Autodesk Inventor part; units mm, degrees
ref_plane "YZ Plane" through (0, 0, 0) normal (1, 0, 0) x (0, 1, 0)
ref_plane "XZ Plane" through (0, 0, 0) normal (0, 1, 0) x (-1, 0, 0)
ref_plane "XY Plane" through (0, 0, 0) normal (0, 0, 1) x (1, 0, 0)
sketch "Sketch1" plane through (0, 0, 0) normal (0, 0, 1) x (1, 0, 0)
  line L0 (0, 0) -> (8.7313, 0) construction
  line L1 (0, 0) -> (0, 7.9375) construction
  line L2 (0, 7.9375) -> (8.7312, 7.9375) construction
  line L3 (8.7312, 7.9375) -> (8.7313, 0) construction
  line L4 (8.7312, 7.9375) -> (47.625, 7.9375) construction
  line L5 (8.7312, 7.9375) -> (8.7312, 14.2875) construction
  line L6 (8.7312, 14.2875) -> (11.9062, 14.2875) construction
  line L7 (11.9062, 14.2875) -> (11.9062, 0) construction
  line L8 (11.9062, 0) -> (8.7313, 0) construction
  line L9 (11.9062, 0) -> (21.4312, 0) construction
  line L10 (21.4312, 0) -> (21.4312, 26.67) construction
  line L11 (21.4312, 26.67) -> (11.9063, 26.67) construction
  line L12 (11.9063, 26.67) -> (11.9062, 14.2875) construction
  line L13 (16.6687, 0) -> (16.6687, 26.67) construction
  line L14 (16.6687, 17.4625) -> (23.8125, 17.4625) construction
  line L15 (23.8125, 17.4625) -> (23.8125, 0) construction
  line L16 (23.8125, 0) -> (21.4312, 0) construction
  line L17 (23.8125, 0) -> (24.6062, 0) construction
  line L18 (24.6062, 0) -> (24.6062, 14.2875) construction
  line L19 (24.6062, 14.2875) -> (23.8125, 14.2875) construction
  line L20 (23.8125, 14.2875) -> (23.8125, 0) construction
  line L21 (24.6062, 0) -> (34.1312, 0) construction
  line L22 (34.1312, 0) -> (34.1313, 20.32) construction
  line L23 (34.1313, 20.32) -> (24.6062, 20.32) construction
  line L24 (24.6062, 20.32) -> (24.6062, 0) construction
  line L25 (29.3687, 20.32) -> (29.3687, 0) construction
  line L26 (29.3687, 17.4625) -> (36.5125, 17.4625) construction
  line L27 (36.5125, 17.4625) -> (36.5125, 0) construction
  line L28 (36.5125, 0) -> (34.1312, 0) construction
  line L29 (36.5125, 0) -> (37.3062, 0) construction
  line L30 (37.3062, 0) -> (37.3062, 14.2875) construction
  line L31 (37.3062, 14.2875) -> (36.5125, 14.2875) construction
  line L32 (36.5125, 14.2875) -> (36.5125, 0) construction
  line L33 (37.3062, 0) -> (38.8937, 0) construction
  line L34 (38.8937, 0) -> (38.8937, 9.525) construction
  line L35 (38.8937, 9.525) -> (37.3062, 9.525) construction
  line L36 (37.3062, 9.525) -> (37.3062, 0) construction
  line L37 (47.625, 7.9375) -> (47.625, 0) construction
  line L38 (47.625, 0) -> (38.8937, 0) construction
  line L39 (14.2875, 26.67) -> (14.2875, 0) construction
  line L40 (26.9875, 20.32) -> (26.9875, 0) construction
  line L41 (0, 7.9375) -> (0, 17.4625) construction
  line L42 (0, 17.4625) -> (8.7312, 17.4625) construction
  line L43 (8.7312, 17.4625) -> (8.7312, 14.2875) construction
  line L44 (0, 3.175) -> (47.625, 3.175) construction
  circle A0 centre (14.2875, 5.5563) radius 2.3813 construction
  circle A1 centre (26.9875, 5.5562) radius 2.3812 construction
  circle A2 centre (14.2875, 5.8102) radius 2.3813 construction
  circle A3 centre (14.2875, 7.5565) radius 2.3813 construction
  circle A4 centre (26.9875, 5.8103) radius 2.3812 construction
  circle A5 centre (26.9875, 7.5565) radius 2.3812 construction
  line L45 (11.9062, 8.1915) -> (16.6687, 8.1915) construction
  line L46 (15.0198, 3.175) -> (17.0201, 5.1753) construction
  line L47 (17.0201, 5.1753) -> (24.2549, 5.1753) construction
  line L48 (24.2549, 5.1753) -> (26.2552, 3.175) construction
  line L49 (24.6062, 8.1915) -> (29.3687, 8.1915) construction
  line L50 (12.7, 5.1753) -> (19.8713, 5.1753) construction
  line L51 (28.575, 5.1753) -> (21.4037, 5.1753)
  line L52 (0, 6.35) -> (9.1122, 6.35) construction
  line L53 (9.1122, 6.35) -> (9.1122, 0) construction
  line L54 (12.7, 5.1753) -> (10.6997, 3.175) construction
  line L55 (19.8713, 5.1753) -> (21.8716, 3.175) construction
  line L56 (21.8716, 3.175) -> (28.575, 3.175) construction
  line L57 (28.575, 3.175) -> (30.4827, 0) construction
  line L58 (28.575, 5.1753) -> (30.5753, 3.175)
  line L59 (30.5753, 3.175) -> (37.2787, 3.175)
  line L60 (37.2787, 3.175) -> (39.1864, 0)
  line L61 (9.1122, 5.5562) -> (47.625, 5.5563) construction
  line L62 (39.5833, 0) -> (36.2448, 5.5563) construction
  line L63 (21.4037, 5.1753) -> (19.4034, 3.175)
  line L64 (19.4034, 3.175) -> (-3.0861, 3.175)
  line L65 (47.625, 7.9375) -> (47.625, 17.4625) construction
  line L66 (47.625, 17.4625) -> (38.8937, 17.4625) construction
  line L67 (38.8937, 17.4625) -> (38.8937, 9.525) construction
  line L68 (47.625, 7.9375) -> (53.975, 7.9375) construction
  line L69 (53.975, 7.9375) -> (53.975, 0) construction
  line L70 (53.975, 0) -> (47.625, 0) construction
  line L71 (53.975, 6.35) -> (66.675, 6.35) construction
  line L72 (66.675, 6.35) -> (66.675, 0) construction
  line L73 (66.675, 0) -> (53.975, 0) construction
  line L74 (-8.0645, 3.175) -> (-8.0645, 2.3812) construction
  line L75 (-8.0645, 0) -> (39.1864, 0)
  line L76 (-3.0861, 3.175) -> (-3.0861, 2.3812)
  line L77 (-3.0861, 2.3812) -> (-8.0645, 2.3812)
  line L78 (-8.0645, 3.175) -> (-8.0645, 6.35) construction
  line L79 (-8.0645, 6.35) -> (-3.0861, 6.35) construction
  line L80 (-3.0861, 6.35) -> (-3.0861, 3.175) construction
  line L81 (-3.0861, 0) -> (-3.0861, 2.3812) construction
  line L82 (-1.5875, 0) -> (-1.5875, 11.1125) construction
  line L83 (-1.5875, 11.1125) -> (-3.0861, 11.1125) construction
  line L84 (-3.0861, 11.1125) -> (-3.0861, 6.35) construction
  line L85 (-3.0861, 3.175) -> (-8.0645, 3.175) construction
  line L86 (-8.0645, 2.3812) -> (-8.0645, 0) construction
  line L87 (-8.0645, 2.7051) -> (-9.5631, 2.7051) construction
  line L88 (-9.5631, 2.7051) -> (-9.5631, 0) construction
  line L89 (-9.5631, 0) -> (-8.0645, 0) construction
  line L90 (-8.0645, 1.4224) -> (-5.5245, 1.4224) construction
  line L91 (-5.5245, 1.4224) -> (-5.5245, 0) construction
  line L92 (-5.5245, 1.4224) -> (-2.9845, 1.4224) construction
  line L93 (-2.9845, 1.4224) -> (-2.9845, 0) construction
  line L94 (-3.0861, 11.1125) -> (-14.2875, 11.1125) construction
  line L95 (-14.2875, 11.1125) -> (-14.2875, 5.9531) construction
  line L96 (-14.2875, 5.9531) -> (-18.4912, 5.9531) construction
  line L97 (-18.4912, 5.9531) -> (-18.4912, 0) construction
  line L98 (-18.4912, 0) -> (-9.5631, 0) construction
  line L99 (-8.0645, 3.9687) -> (-14.5224, 3.9687) construction
  line L100 (-14.5224, 3.9687) -> (-14.5224, 0) construction
  line L101 (-14.5224, 3.429) -> (-10.3568, 3.429) construction
  line L102 (-10.3568, 3.429) -> (-10.3568, 0) construction
  line L103 (-16.9037, 3.175) -> (-16.9037, 0) construction
  line L104 (-16.9037, 3.175) -> (-18.4912, 3.175) construction
  dimension "d0" = 8.7312
  dimension "d1" = 7.9375
  dimension "d2" = 3.175
  dimension "d3" = 14.2875
  dimension "d4" = 9.525
  dimension "d5" = 26.67
  dimension "d6" = 7.1437
  dimension "d7" = 17.4625
  dimension "d8" = 0.7937
  dimension "d9" = 14.2875
  dimension "d10" = 9.525
  dimension "d11" = 20.32
  dimension "d12" = 7.1437
  dimension "d13" = 17.4625
  dimension "d14" = 0.7937
  dimension "d15" = 14.2875
  dimension "d16" = 1.5875
  dimension "d17" = 9.525
  dimension "d18" = 8.7312
  dimension "d19" = 2.3813
  dimension "d20" = 2.3813
  dimension "d21" = 17.4625
  dimension "d22" = 3.175
  dimension "d23" = 4.7625
  dimension "d24" = 4.7625
  dimension "d26" = 0.254
  dimension "d28" = 45
  dimension "d29" = 45
  dimension "d30" = 0.254
  dimension "d31" = 7.2348
  dimension "d32" = 5.1753
  dimension "d33" = 7.1713
  dimension "d34" = 1.5875
  dimension "d35" = 7.1713
  dimension "d36" = 1.5875
  dimension "d37" = 6.35
  dimension "d39" = 45
  dimension "d40" = 45
  dimension "d41" = 1.5875
  dimension "d42" = 59
  dimension "d43" = 6.7034
  dimension "d44" = 6.7034
  dimension "d45" = 5.5563
  dimension "d46" = 0.3969
  dimension "d47" = 1.5875
  dimension "d48" = 9.1122
  dimension "d52" = 17.4625
  dimension "d53" = 6.35
  dimension "d54" = 12.7
  dimension "d55" = 6.35
  dimension "d56" = 2.3813
  dimension "d57" = 4.9784
  dimension "d58" = 6.35
  dimension "d66" = 1.4986
  dimension "d67" = 1.5875
  dimension "d68" = 11.1125
  dimension "d69" = 2.7051
  dimension "d70" = 1.4986
  dimension "d71" = 1.4224
  dimension "d72" = 2.54
  dimension "d73" = 2.54
  dimension "d74" = 3.9688
  dimension "d75" = 4.1656
  dimension "d76" = 3.429
sketch "Sketch2" plane through (0, 0, 0) normal (0, 0, 1) x (1, 0, 0)
  line L0 (19.4034, 3.175) -> (-3.0861, 3.175)
  line L1 (-3.0861, 3.175) -> (-3.0861, 2.3812)
  line L2 (-3.0861, 2.3812) -> (-8.0645, 2.3812)
  line L3 (-8.0645, 2.3812) -> (-8.0645, 0)
  line L4 (-8.0645, 0) -> (39.1864, 0)
  line L5 (37.2787, 3.175) -> (39.1864, 0)
  line L6 (30.5753, 3.175) -> (37.2787, 3.175)
  line L7 (28.575, 5.1753) -> (30.5753, 3.175)
  line L8 (28.575, 5.1753) -> (21.4037, 5.1753)
  line L9 (21.4037, 5.1753) -> (19.4034, 3.175)
  point P0 (0, 0)
revolve "Revolution1" add sketch "Sketch2" angle 360 about axis through (-8.0645, 0, 0) along (1, 0, 0)
sketch "Sketch3" plane through (-8.0645, 0, 0) normal (-1, 0, 0) x (0, 0, 1)
  circle A0 centre (0, 0) radius 2.3813
hole "Hole1" at (-8.0645, 0, 0) direction (1, 0, 0) diameter 2.159 depth 3.81 tip angle 118
equation "\"d9\" = d3"
equation "\"d12\" = d6"
equation "\"d13\" = d7"
equation "\"d15\" = d9"
equation "\"d18\" = d0"
equation "\"d20\" = d19"
equation "\"d35\" = d33"
equation "\"d36\" = d34"
equation "\"d43\" = d44"
equation "\"d52\" = d13"
properties part number "Ball Shifting Outline" material "Steel, Alloy"
Input: part model. Units: mm. Frame: model coordinates. A direction names the side the tool comes from. Give positions to 0.01 mm unless a question says otherwise; leave off trailing zeros. Write each loop counter-clockwise with the first axis right and the second up, starting at its lowest first coordinate (ties: lowest second). Pieces come first, ordered by that corner, then holes. Notation, with made-up numbers: M 10.5,60.25 L 58.5,60.25 A10 ccw 58.5,76.25 Z; hole C -5.75,17.25 d6. An arc over 180 degrees is marked long. Write item = value, one per line. Start each with the question number.
1) Reachability of faces 1 (the cylindrical face through (-5.61, -0.516, 2.325)), 2 (the cylindrical face through (24.94, -0.67, -5.13)), 3 (the cylindrical face through (33.97, -0.69, -3.1)) from +Z, -Z, +X, -X, +Y, -Y: full face, straight path, thin tool, end or side. Return the list, or none.
2) Draft query along Y for faces 4 (the flat face through (-8.065, 1, 1)), 5 (the cylindrical face through (-6.13, -1.07, -0.14)), 6 (the cylindrical face through (8, -0.69, 3.1)), 7 (the conical face through (-3.719, -0.183, -0.041)). Return one class per face: +Y half, -Y half, draft (parallel to the pull), parting line (faces both ways), or undercut.
3) Cut plane A-A on x = 12. Return the cut outline in (y, z) (3 decimals), then the cut area to 3 significant figures.
4) Material intervals for line 1 along Z through (x, y) = (-5.6, 0); line 2 along X through (y, z) = (-3.5, -3); line 3 along Z through (x, y) = (10.5, 1.5), sorted ascending. Write a range as [from, to].
5) First-contact query: pin 1 Ø3 at (x, z) = (25.5, -1.5) entering from +Y; pin 2 Ø3 at (x, z) = (23.5, -3) entering from -Y; pin 3 Ø1.5 at (y, z) = (0.5, 1) entering from +X; pin 4 Ø4 at (x, z) = (5, -1.5) entering from -Y (3 decimals). Flat tips, straight axial feed; report the tip coordinate or a pass-through.
Solved:
q1.face_1 = -X
q1.face_2 = +X, -X
q1.face_3 = +X
q2.face_4 = draft
q2.face_5 = undercut
q2.face_6 = parting line
q2.face_7 = undercut
q3.outline = C 0,0 d6.35
q3.area = 31.7 mm2
q4.line_1 = [-2.38, -1.08], [1.08, 2.38]
q4.line_2 = [20.84, 29.14]
q4.line_3 = [-2.8, 2.8]
q5.pin_1 = 5.18
q5.pin_2 = -4.95
q5.pin_3 = 38.97
q5.pin_4 = -3.175
